CAD build for the part. Positions are in the model's coordinates, mm. Give positions to 0.01 mm unless a question says otherwise; leave off trailing zeros. Loops run counter-clockwise (first coordinate to the right, second up) from the corner with the lowest first, then second, coordinate; pieces in that order, holes last. Notation, with made-up numbers: (76, -25.5) -> (93, -25.5) arc R25 cw to (93, 10.5) -> close; hole circle Ø4 at (35, 6.25). An arc over 180 degrees is marked (long way). Use one line per item in the form item = value.
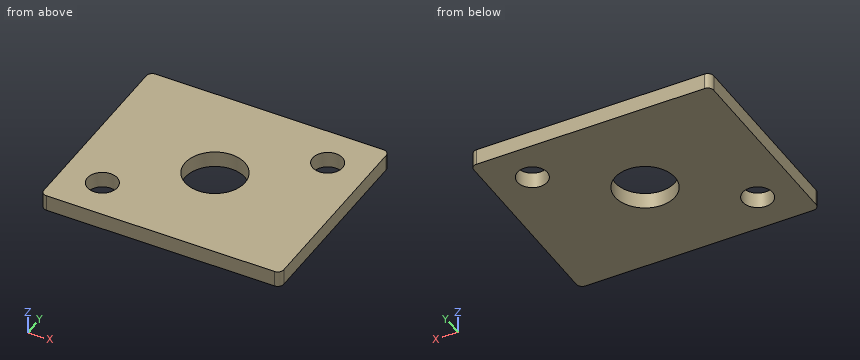
```python
from build123d import *

# Parameters (mm, degrees)
SKIZZE1_W                       = 12
SKIZZE1_H                       = 10
AUFSATZ_LINEAR_AUSTRAGEN1_DEPTH = 0.8
SKIZZE2_R                       = 0.75
SKIZZE2_R_2                     = 1.5
SCHNITT_LINEAR_AUSTRAGEN1_DEPTH = 16.640971837
VERRUNDUNG1_R                   = 0.3


with BuildPart() as part:
    # Skizze1 → Aufsatz-Linear austragen1 (new body)
    with BuildSketch(Plane.XY):
        with Locations((6, 5)):
            Rectangle(SKIZZE1_W, SKIZZE1_H)
    extrude(amount=AUFSATZ_LINEAR_AUSTRAGEN1_DEPTH)

    # Skizze2 → Schnitt-Linear austragen1 (cut, through all)
    with BuildSketch(Plane.XY.offset(0.8)):
        with Locations((2, 2)):
            Circle(SKIZZE2_R)
        with Locations((6, 5)):
            Circle(SKIZZE2_R_2)
        with Locations((10, 8)):
            Circle(SKIZZE2_R)
    extrude(amount=-SCHNITT_LINEAR_AUSTRAGEN1_DEPTH, mode=Mode.SUBTRACT)

    # Verrundung1
    verrundung1_edges = [part.edges().sort_by_distance(p)[0] for p in [
        (0, 10, 0.4),
        (12, 10, 0.4),
        (12, 0, 0.4),
        (0, 0, 0.4),
    ]]
    fillet(verrundung1_edges, radius=VERRUNDUNG1_R)


solid = part.part
```
1. Drop a flat-ended pin along its axis: P1, Ø1.2, axis at x = 2, y = 2, coming from the +Z side. Give the stop position or say it passes through.
Result sheet:
P1 = through
2. Cut at B-B, the plane z = 0.2. Write the cut outline in (x, y), then the cut area to 3 significant figures.
Result sheet:
outline = (0, 0.3) arc R0.3 ccw to (0.3, 0) -> (11.7, 0) arc R0.3 ccw to (12, 0.3) -> (12, 9.7) arc R0.3 ccw to (11.7, 10) -> (0.3, 10) arc R0.3 ccw to (0, 9.7) -> close; hole circle Ø1.5 at (2, 2); hole circle Ø3 at (6, 5); hole circle Ø1.5 at (10, 8)
area = 109 mm^2
3. Cut at C-C, the plane x = 6. Write the cut outline in (y, z), then the cut area to 3 significant figures.
Result sheet:
outline = (0, 0) -> (3.5, 0) -> (3.5, 0.8) -> (0, 0.8) -> close; (6.5, 0) -> (10, 0) -> (10, 0.8) -> (6.5, 0.8) -> close
area = 5.60 mm^2
4. Drill centre lines: line 1 (Y direction, x = 10, z = 0.2); line 2 (Y direction, x = 2, z = 0.65); line 3 (X direction, y = 1.75, z = 0.3). Where is each one in solid material? Low to high.
Result sheet:
line_1 = 0 to 7.25, 8.75 to 10
line_2 = 0 to 1.25, 2.75 to 10
line_3 = 0 to 1.29, 2.71 to 12
5. Cut at A-A, the plane y = 2. Write the cut outline in (x, z), then the cut area to 3 significant figures.
Result sheet:
outline = (0, 0) -> (1.25, 0) -> (1.25, 0.8) -> (0, 0.8) -> close; (2.75, 0) -> (12, 0) -> (12, 0.8) -> (2.75, 0.8) -> close
area = 8.40 mm^2
